```python
from build123d import *

# Parameters (mm, degrees)
SKETCH1_W                  = 25.4
SKETCH1_H                  = 63.5
SKETCH1_R                  = 2.0701
SKETCH1_R_2                = 3.175
BASE_FLANGE1_DEPTH         = 2.54
SKETCHED_START             = -25.4
SKETCHED_BEND1_DEPTH       = 25.4
SKETCHED_START_2           = -15.8749999
SKETCHED_BEND1_2_DEPTH     = 15.8749999
SKETCHED_BEND1_3_DEPTH     = 3.1749999
SKETCHED_START_3           = -22.2250001
SKETCHED_BEND1_4_DEPTH     = 6.3500002
SKETCHED_START_4           = 10.884911335
SKETCHED_BEND1_5_OUTLINE_R = 3.175
SKETCHED_BEND1_5_DEPTH     = 2.54
FILLET1_R                  = 12.7
FILLET2_R                  = 2.54


with BuildPart() as part:
    # Base-Flange1: sheet metal written as solids
    # Sketch1 → Base-Flange1 (new body)
    with BuildSketch(Plane.XY):
        with Locations((-12.7, 31.75)):
            Rectangle(SKETCH1_W, SKETCH1_H)
        with Locations((-12.7, 50.8)):
            Circle(SKETCH1_R, mode=Mode.SUBTRACT)
        with Locations((-19.05, 6.35)):
            Circle(SKETCH1_R_2, mode=Mode.SUBTRACT)
    extrude(amount=-BASE_FLANGE1_DEPTH)

    # Sketched Bend1: read off the stored shape, not the designer's step
    # Sketched Bend1 outline → Sketched Bend1 (cut)
    with BuildSketch(Plane.YZ.offset(SKETCHED_START)):
        with BuildLine():
            ThreePointArc((14.694911335, -2.54), (12.49520681, -1.840851973), (11.102808887, 0))
            Line((11.102808887, 0), (0, 0))
            Line((0, 0), (0, -2.54))
            Line((0, -2.54), (14.694911335, -2.54))
        make_face()
    extrude(amount=SKETCHED_BEND1_DEPTH, mode=Mode.SUBTRACT)

    # Sketched Bend1 2 outline → Sketched Bend1 2 (add)
    with BuildSketch(Plane.YZ.offset(SKETCHED_START_2)):
        with BuildLine():
            Line((10.884911335, 11.975088665), (10.884911335, 1.27))
            ThreePointArc((10.884911335, 1.27), (10.939780823, 0.625721461), (11.102808887, 0))
            Line((11.102808887, 0), (14.694911335, 0))
            ThreePointArc((14.694911335, 0), (13.796885723, 0.371974388), (13.424911335, 1.27))
            Line((13.424911335, 1.27), (13.424911335, 11.975088665))
            Line((13.424911335, 11.975088665), (10.884911335, 11.975088665))
        make_face()
    extrude(amount=SKETCHED_BEND1_2_DEPTH)

    # Sketched Bend1 3 outline → Sketched Bend1 3 (add)
    with BuildSketch(Plane.YZ.offset(SKETCHED_START)):
        with BuildLine():
            Line((10.884911335, 11.975088665), (10.884911335, 1.27))
            ThreePointArc((10.884911335, 1.27), (10.939780823, 0.625721461), (11.102808887, 0))
            Line((11.102808887, 0), (14.694911335, 0))
            ThreePointArc((14.694911335, 0), (13.796885723, 0.371974388), (13.424911335, 1.27))
            Line((13.424911335, 1.27), (13.424911335, 11.975088665))
            Line((13.424911335, 11.975088665), (10.884911335, 11.975088665))
        make_face()
    extrude(amount=SKETCHED_BEND1_3_DEPTH)

    # Sketched Bend1 4 outline → Sketched Bend1 4 (add)
    with BuildSketch(Plane.YZ.offset(SKETCHED_START_3)):
        with BuildLine():
            Line((10.884911335, 11.975088665), (10.884911335, 1.27))
            ThreePointArc((10.884911335, 1.27), (10.939780823, 0.625721461), (11.102808887, 0))
            Line((11.102808887, 0), (14.694911335, 0))
            ThreePointArc((14.694911335, 0), (13.796885723, 0.371974388), (13.424911335, 1.27))
            Line((13.424911335, 1.27), (13.424911335, 11.975088665))
            Line((13.424911335, 11.975088665), (10.884911335, 11.975088665))
        make_face()
    extrude(amount=SKETCHED_BEND1_4_DEPTH)

    # Sketched Bend1 5 outline → Sketched Bend1 5 (cut)
    with BuildSketch(Plane(origin=(0, 0, 0), x_dir=(1, 0, 0), z_dir=(0, 1, 0)).offset(SKETCHED_START_4)):
        with Locations((-19.05, -5.625088665)):
            Circle(SKETCHED_BEND1_5_OUTLINE_R)
    extrude(amount=SKETCHED_BEND1_5_DEPTH, mode=Mode.SUBTRACT)

    # Fillet1
    fillet1_edges = [part.edges().sort_by_distance(p)[0] for p in [
        (-25.4, 63.5, -1.27),
        (0, 63.5, -1.27),
    ]]
    fillet(fillet1_edges, radius=FILLET1_R - 0.0001)  # a hair under: the kernel refuses the full size

    # Fillet2
    fillet2_edges = [part.edges().sort_by_distance(p)[0] for p in [
        (0, 12.154911335, 11.975088665),
        (-25.4, 12.154911335, 11.975088665),
    ]]
    fillet(fillet2_edges, radius=FILLET2_R)


solid = part.part
```
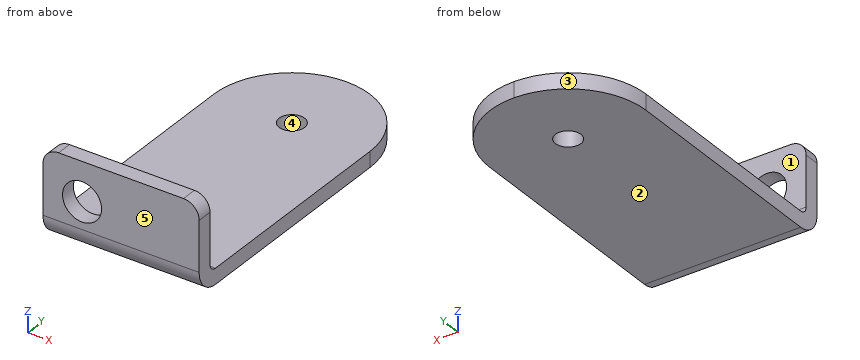
For this review, take the finished solid that the model builds, in its own axes (mm). Face numbers are marked on the shaded views. A direction names the side the tool comes from. Round coordinates to 2 decimals unless told otherwise and drop trailing zeros. Write each loop counter-clockwise with the first axis right and the second up, starting at its lowest first coordinate (ties: lowest second). Pieces come first, ordered by that corner, then holes. Notation, with made-up numbers: (21.5, 60) -> (50.5, 60) arc R19 ccw to (50.5, 83) -> close; hole circle Ø11 at (-19, 78.25). An arc over 180 degrees is marked (long way). One line per question, with ' | ' between items. Start each with the question number.
(1) Insertion check: P1, Ø5, axis at x = -5.5, y = 25.5, coming from the +Z side; P2, Ø7.5, axis at x = -19.05, z = 5.63, coming from the +Y side; P3, Ø1.5, axis at x = -11.5, z = -1, coming from the +Y side; P4, Ø5, axis at x = -12.7, y = 50.8, coming from the -Z side. Each pin has a flat end and moves straight along its axis. Give the tip position at first contact, or say it passes through.
(2) Mouldability with a two-part tool opening along X and no side actions: class the marked faces 3, 4 and 5 as released by +X, released by -X, zero draft, split by the parting line, or undercut.
(3) For line 1 along Y through (x, z) = (-12.25, 2.25); line 2 along Z through (x, y) = (-1.25, 16.5); line 3 along Z through (x, y) = (-19.05, 12.7), list the stretches that pass through material, from the lowest coordinate up. Write a range as from..to.
(4) Add section C-C, the plane y = 19. Write out the cut boundary in (x, z), plus the area to 3 significant figures.
(5) Tool access review of the marked faces 1 and 2: name each direction out of +Z, -Z, +X, -X, +Y, -Y from which nothing blocks a thin tool from reaching the whole face with its end or side.
(6) Add section A-A, the plane x = -19.05. Write out the cut boundary in (y, z), plus the area to 3 significant figures.
(7) Add section B-B, the plane x = -2. Write out the cut boundary in (y, z), plus the area to 3 significant figures.
(8) Add section D-D, the plane x = -13.5. Write out the cut boundary in (y, z).
Answer list:
1) P1: z = 0 | P2: y = 13.42 | P3: y = 63.49 | P4: z = -2.54
2) face 3: released by -X | face 4: undercut | face 5: zero draft
3) line 1: 10.88..13.42 | line 2: -2.54..0 | line 3: -1.98..2.45, 8.8..11.98
4) outline: (-25.4, -2.54) -> (0, -2.54) -> (0, 0) -> (-25.4, 0) -> close | area: 64.5 mm²
5) face 1: +Z, +X, -X, +Y | face 2: -Z, +X, -X, +Y, -Y
6) outline: (10.88, 1.27) arc R3.81 ccw to (14.69, -2.54) -> (61.8, -2.54) -> (61.8, 0) -> (14.69, 0) arc R1.27 cw to (13.42, 1.27) -> (13.42, 2.45) -> (10.88, 2.45) -> close; (10.88, 8.8) -> (13.42, 8.8) -> (13.42, 11.98) -> (10.88, 11.98) -> close | area: 141 mm²
7) outline: (10.88, 1.27) arc R3.81 ccw to (14.69, -2.54) -> (57.64, -2.54) -> (57.64, 0) -> (14.69, 0) arc R1.27 cw to (13.42, 1.27) -> (13.42, 11.92) -> (10.88, 11.92) -> close | area: 146 mm²
8) outline: (10.88, 1.27) arc R3.81 ccw to (14.69, -2.54) -> (48.89, -2.54) -> (48.89, 0) -> (14.69, 0) arc R1.27 cw to (13.42, 1.27) -> (13.42, 11.98) -> (10.88, 11.98) -> close; (52.71, -2.54) -> (63.47, -2.54) -> (63.47, 0) -> (52.71, 0) -> close
